Design review of the part built by this model. Coordinates are the model's own, in mm. Face numbers are marked on the shaded views. A direction names the side the tool comes from. Coordinates: 2 decimals unless noted, no trailing zeros. Write item = value, one per line. Start each with the question number.
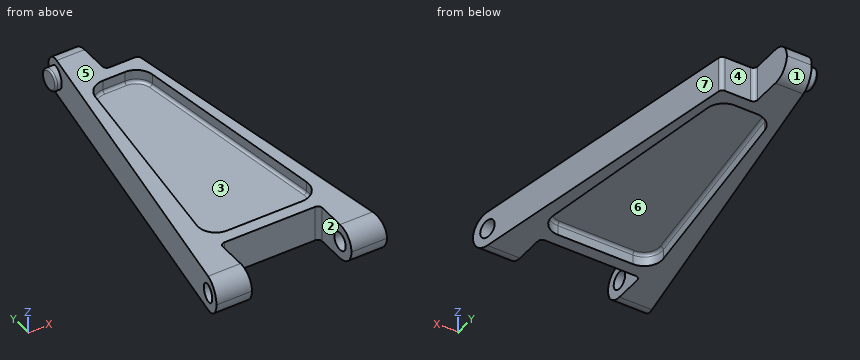
```python
from build123d import *

# Parameters (mm, degrees)
BOSS_EXTRUDE1_DEPTH     = 50
FILLET1_R               = 50
CUT_EXTRUDE2_DEPTH      = 1030.611577246
CUT_EXTRUDE2_DEPTH_BACK = 1030.611577246
SKETCH4_W               = 280
SKETCH4_H               = 140
SKETCH4_W_2             = 94
SKETCH5_R               = 30
BOSS_EXTRUDE2_DEPTH     = 100
FILLET2_R               = 5
FILLET3_R               = 12
CUT_EXTRUDE4_DEPTH      = 35
FILLET4_R               = 50
FILLET5_R               = 8
FILLET4_OF_MIRROR1_R    = 50
FILLET5_OF_MIRROR1_R    = 8
SKETCH7_R               = 25
CUT_EXTRUDE5_DEPTH      = 250


with BuildPart() as part:
    # Sketch1 → Boss-Extrude1 (new, symmetric)
    with BuildSketch(Plane.XY):
        Polygon((-240, 0), (240, 0), (70, 1000), (-70, 1000), align=None)
    extrude(amount=BOSS_EXTRUDE1_DEPTH, both=True)

    # Fillet1
    fillet1_edges = [part.edges().sort_by_distance(p)[0] for p in [
        (0, 1000, 50),
        (0, 1000, -50),
        (0, 0, 50),
        (0, 0, -50),
    ]]
    fillet(fillet1_edges, radius=FILLET1_R - 0.0001)  # a hair under: the kernel refuses the full size

    # Sketch4 → Cut-Extrude2 (cut, two sides: drawn at the far end of the back side and taken through both)
    with BuildSketch(Plane.XY.offset(-CUT_EXTRUDE2_DEPTH_BACK)):
        with Locations((0, 70)):
            Rectangle(SKETCH4_W, SKETCH4_H)
        with Locations((47, 930)):
            Rectangle(SKETCH4_W_2, SKETCH4_H)
    extrude(amount=CUT_EXTRUDE2_DEPTH + CUT_EXTRUDE2_DEPTH_BACK, mode=Mode.SUBTRACT)

    # Sketch5 → Boss-Extrude2 (add)
    with BuildSketch(Plane(origin=(0, 0, 0), x_dir=(0, 0, -1), z_dir=(1, 0, 0))):
        with Locations((0, 950)):
            Circle(SKETCH5_R)
    extrude(amount=-BOSS_EXTRUDE2_DEPTH)

    # Fillet2
    fillet2_edges = [part.edges().sort_by_distance(p)[0] for p in [
        (-100, 950, 30),
    ]]
    fillet(fillet2_edges, radius=FILLET2_R)

    # Fillet3
    fillet3_edges = [part.edges().sort_by_distance(p)[0] for p in [
        (-140, 140, 0),
        (140, 140, 0),
        (93.8, 860, 0),
        (0, 860, 0),
    ]]
    fillet(fillet3_edges, radius=FILLET3_R)

    # Sketch6 → Cut-Extrude4 (cut)
    with BuildSketch(Plane.XY.offset(50)):
        Polygon((76.441272438, 825), (-72.757259745, 825), (-153.811728433, 175), (171.475101543, 175), align=None)
    cut_extrude4 = extrude(amount=-CUT_EXTRUDE4_DEPTH, mode=Mode.SUBTRACT)

    # Fillet4
    fillet4_edges = [part.edges().sort_by_distance(p)[0] for p in [
        (76.441272438, 825, 32.5),
        (171.475101543, 175, 32.5),
        (-153.811728433, 175, 32.5),
        (-72.757259745, 825, 32.5),
    ]]
    fillet(fillet4_edges, radius=FILLET4_R)

    # Fillet5
    fillet5_edges = [part.edges().sort_by_distance(p)[0] for p in [
        (122.900622431, 507.233392258, 15),
        (8.221853466, 175, 15),
        (2.307508674, 825, 15),
        (-112.512975158, 506.187040802, 15),
        (-61.700650501, 812.479007725, 15),
        (65.918080265, 812.826377126, 15),
        (-134.668529482, 191.904320827, 15),
        (151.459605814, 192.301908411, 15),
    ]]
    fillet(fillet5_edges, radius=FILLET5_R)

    # Mirror1: Cut-Extrude4 across plane
    add(cut_extrude4.mirror(Plane.XY), mode=Mode.SUBTRACT)

    # Fillet4 of Mirror1
    fillet4_of_mirror1_edges = [part.edges().sort_by_distance(p)[0] for p in [
        (76.441272438, 825, -32.5),
        (171.475101543, 175, -32.5),
        (-153.811728433, 175, -32.5),
        (-72.757259745, 825, -32.5),
    ]]
    fillet(fillet4_of_mirror1_edges, radius=FILLET4_OF_MIRROR1_R)

    # Fillet5 of Mirror1
    fillet5_of_mirror1_edges = [part.edges().sort_by_distance(p)[0] for p in [
        (122.900622431, 507.233392258, -15),
        (8.221853466, 175, -15),
        (2.307508674, 825, -15),
        (-112.512975158, 506.187040802, -15),
        (-61.700650501, 812.479007725, -15),
        (65.918080265, 812.826377126, -15),
        (-134.668529482, 191.904320827, -15),
        (151.459605814, 192.301908411, -15),
    ]]
    fillet(fillet5_of_mirror1_edges, radius=FILLET5_OF_MIRROR1_R)

    # Sketch7 → Cut-Extrude5 (cut, symmetric)
    with BuildSketch(Plane(origin=(0, 0, 0), x_dir=(0, 0, -1), z_dir=(1, 0, 0))):
        with Locations((0, 50)):
            Circle(SKETCH7_R)
    extrude(amount=CUT_EXTRUDE5_DEPTH, both=True, mode=Mode.SUBTRACT)


solid = part.part
```
(1) Mouldability with a two-part tool opening along Y and no side actions: class the marked faces 5, 6 and 7 as pulls with the +Y half, pulls with the -Y half, needs draft (parallel to the pull), parting line crosses it, or undercut.
(2) For line 1 (Z direction, x = 168, y = 50); line 2 (X direction, y = 789.5, z = 25) (3 decimals); line 3 (X direction, y = 317, z = -40), list the stretches that pass through material, from the lowest coordinate up.
(3) For pin 1 Ø6 at (y, z) = (447, -5.5) entering from -X; pin 2 Ø13.5 at (x, z) = (13.5, -34) entering from +Y; pin 3 Ø8 at (x, z) = (-4, -32) entering from -Y, all flat-tipped, find the tip position at first contact; note any pin that passes through.
(4) For the marked faces 1, 2, 3 and 4, list the 3-axis set-ups (+Z, -Z, +X, -X, +Y, -Y) from which the entire face can be reached by the end or side of a thin tool; tool diameter is ignored.
Report:
q1.face_5 = needs draft
q1.face_6 = undercut
q1.face_7 = pulls with the +Y half
q2.line_1 = -50 to -25, 25 to 50
q2.line_2 = -105.785 to -76.456, 81.071 to 105.785
q2.line_3 = -186.11 to -136.1, 150.71 to 186.11
q3.pin_1 = -164.52
q3.pin_2 = 861.21
q3.pin_3 = 140
q4.face_1 = -Z, +X, -X, +Y
q4.face_2 = +Z, -Z, -Y
q4.face_3 = +Z
q4.face_4 = +Z, -Z, +X, +Y
